Autodesk Inventor part; units mm, degrees
ref_plane "YZ Plane" through (0, 0, 0) normal (1, 0, 0) x (0, 1, 0)
ref_plane "XZ Plane" through (0, 0, 0) normal (0, 1, 0) x (-1, 0, 0)
ref_plane "XY Plane" through (0, 0, 0) normal (0, 0, 1) x (1, 0, 0)
sketch "Sketch1" plane through (0, 0, 0) normal (0, 0, 1) x (1, 0, 0)
  line L0 (-30.75, -46) -> (30.75, -46)
  line L1 (30.75, -46) -> (30.75, 46)
  line L2 (30.75, 46) -> (-30.75, 46)
  line L3 (-30.75, 46) -> (-30.75, -46)
  line L4 (-30.75, -46) -> (30.75, 46) construction
  line L5 (30.75, -46) -> (-30.75, 46) construction
  point P0 (0, 0)
  dimension "d0" = 92
  dimension "d1" = 61.5
extrude "Extrusion1" add sketch "Sketch1" along normal blind 26.4
sketch "Sketch3" plane through (0, 0, 26.4) normal (0, 0, 1) x (1, 0, 0)
  line L0 (-23.375, -34.95) -> (23.375, -34.95) construction
  line L1 (23.375, -34.95) -> (23.375, 34.95) construction
  line L2 (23.375, 34.95) -> (-23.375, 34.95) construction
  line L3 (-23.375, 34.95) -> (-23.375, -34.95) construction
  line L4 (-23.375, -34.95) -> (23.375, 34.95) construction
  line L5 (23.375, -34.95) -> (-23.375, 34.95) construction
  circle A0 centre (-23.375, -34.95) radius 3
  circle A1 centre (23.375, -34.95) radius 3
  circle A2 centre (23.375, 34.95) radius 3
  circle A3 centre (-23.375, 34.95) radius 3
  point P0 (0, 0)
  dimension "d5" = 46.75
  dimension "d6" = 69.9
  dimension "d7" = 6
extrude "Extrusion2" add sketch "Sketch3" along normal blind 4
sketch "Sketch4" plane through (-30.75, 46, 0) normal (0, 1, 0) x (1, 0, 0)
  line L0 (0.1106, -5.25) -> (61.5, -5.25) construction
  line L1 (61.5, 0) -> (61.5, -26.4) construction
  line L2 (61.5, 0) -> (0, 0) construction
  line L3 (0, 0) -> (61.5, 0) construction
  line L4 (4, 0) -> (4, -26.4) construction
  line L5 (61.5, -26.4) -> (0, -26.4) construction
  line L6 (0, 0) -> (0, -26.4) construction
  line L7 (4, -5.25) -> (21.5, -5.25)
  line L8 (21.5, -5.25) -> (21.5, -20.75)
  line L9 (21.5, -20.75) -> (4, -20.75)
  line L10 (4, -20.75) -> (4, -5.25)
  point P0 (30.75, 0)
  dimension "d10" = 5.25
  dimension "d11" = 4
  dimension "d12" = 15.5
  dimension "d13" = 17.5
extrude "Extrusion3" add sketch "Sketch4" along normal blind 10
sketch "Sketch5" plane through (-30.75, 46, 0) normal (0, 1, 0) x (1, 0, 0)
  line L0 (57.5, 0) -> (57.5, -26.4) construction
  line L1 (61.5, -26.4) -> (0, -26.4) construction
  line L2 (61.5, 0) -> (61.5, -26.4) construction
  line L3 (61.5, 0) -> (0, 0) construction
  line L4 (21.5, 0) -> (21.5, -26.4) construction
  line L5 (21.5, -2) -> (57.5, -2) construction
  line L6 (21.5, -5.25) -> (21.5, -20.75) construction
  line L7 (21.5, -19.5) -> (57.5, -19.5) construction
  line L8 (21.5, -2) -> (57.5, -2)
  line L9 (57.5, -2) -> (57.5, -19.5)
  line L10 (57.5, -19.5) -> (21.5, -19.5)
  line L11 (21.5, -19.5) -> (21.5, -2)
  point P0 (30.75, 0)
  dimension "d16" = 4
  dimension "d17" = 40
  dimension "d18" = 2
  dimension "d19" = 19.5
extrude "Extrusion4" add sketch "Sketch5" along normal blind 10
properties part number "Vilros Pi Case"
Verification items for the finished model (mm, model axes). A direction names the side the tool comes from. Coordinates: 2 decimals unless noted, no trailing zeros. Order: outer loops, then holes, each group sorted by start corner. A loop starts at its lowest first (then second) coordinate and runs counter-clockwise, first axis right, second up. Notation, with made-up numbers: M 30.25,61.25 L 58.25,61.25 A25 ccw 58.25,98.25 Z; hole C 5,5 d2. An arc over 180 degrees is marked long. One line per item, written item: value. Start each with the question number.
Item 1: Scan lines: probe 1 along Z at (x, y) = (8.5, -13); probe 2 along Y at (x, z) = (25.5, 28); probe 3 along Y at (x, z) = (-15, 21). Record each from-to range of solid material in increasing order.
Item 2: Sectioned sample at C-C (z = 28). Enter the section's corners in (x, y) (3 decimals).
Item 3: Sectioned sample at B-B (y = 34.95). Enter the section's corners in (x, z) (3 decimals).
Item 4: Access from +Z, -Z, +X, -X, +Y, -Y to the whole of each face (thin tool, end or side, straight path). Record for faces 1 (the cylindrical face through (21.164, -36.978, 28.372)), 2 (the flat face through (-18, 51, 5.25)), 3 (the flat face through (26.75, 51, 11)).
Item 5: Sectioned sample at A-A (x = 11.5). Enter the section's corners in (y, z), then the cut area to 3 significant figures.
Item 6: Gauge pin test, flat ends, axial feed: pin 1 (11 mm diameter, centred on x = -19, y = 52, fed in from +Z); pin 2 (3 mm diameter, centred on x = -9.5, y = -33, fed in from +Z); pin 3 (1.4 mm diameter, centred on y = 51, z = 20, fed in from +X). Record the tip position at first contact, or that the pin passes through.
Item 7: Sectioned sample at D-D (y = -5). Enter the section's corners in (x, z), then the cut area to 3 significant figures.
Conclusion:
1. probe 1: z = 0 to 26.4
1. probe 2: y = -37.07 to -32.83, 32.83 to 37.07
1. probe 3: y = -46 to 46
2. outline: C -23.375,-34.95 d6; C -23.375,34.95 d6; C 23.375,-34.95 d6; C 23.375,34.95 d6
3. outline: M -30.75,0 L 30.75,0 L 30.75,26.4 L 26.375,26.4 L 26.375,30.4 L 20.375,30.4 L 20.375,26.4 L -20.375,26.4 L -20.375,30.4 L -26.375,30.4 L -26.375,26.4 L -30.75,26.4 Z
4. face 1: +Z
4. face 2: -Z, -X, +Y
4. face 3: +Z, -Z, +X, +Y
5. outline: M -46,0 L 46,0 L 46,2 L 56,2 L 56,19.5 L 46,19.5 L 46,26.4 L -46,26.4 Z
5. area: 2,600 mm^2
6. pin 1: stops at z = 20.75
6. pin 2: stops at z = 26.4
6. pin 3: stops at x = 26.75
7. outline: M -30.75,0 L 30.75,0 L 30.75,26.4 L -30.75,26.4 Z
7. area: 1,620 mm^2
